For this review, take the finished solid that the model builds, in its own axes (mm). A direction names the side the tool comes from. Coordinates: 2 decimals unless noted, no trailing zeros. Loops run counter-clockwise (first coordinate to the right, second up) from the corner with the lowest first, then second, coordinate; pieces in that order, holes last. Notation, with made-up numbers: (25, 28.25) -> (40, 28.25) arc R30 ccw to (40, 56.25) -> close; hole circle Ø10 at (-3, -38.5). An arc over 180 degrees is marked (long way). One line per item, written item: value.
from build123d import *

# Parameters (mm, degrees)
EXTRUDE_1_DEPTH     = 3
SKETCH_2_W          = 12
SKETCH_2_H          = 12
EXTRUDE_2_DEPTH     = 3.5
SKETCH_3_R          = 4.05
EXTRUDE_3_DEPTH     = 15
CUT_EXTRUDE_1_REACH = 58.993
SKETCH_4_R          = 1.4


with BuildPart() as part:
    # Sketch 1 → Extrude 1 (new body)
    with BuildSketch(Plane(origin=(0, 0, 0), x_dir=(0, 0, -1), z_dir=(1, 0, 0))):
        Polygon((-35, -10), (-35, -41), (0, -41), (0, 41), (-35, 41), (-35, 10), (-10, 10), (-10, -10), align=None)
    extrude(amount=EXTRUDE_1_DEPTH)

    # Sketch 2 → Extrude 2 (add)
    with BuildSketch(Plane(origin=(3, 0, 0), x_dir=(0, 0, -1), z_dir=(1, 0, 0))):
        with Locations((-21, -33.5)):
            Rectangle(SKETCH_2_W, SKETCH_2_H)
    extrude_2 = extrude(amount=EXTRUDE_2_DEPTH)

    # Sketch 3 → Extrude 3 (add)
    with BuildSketch(Plane(origin=(6.5, 0, 0), x_dir=(0, 0, -1), z_dir=(1, 0, 0))):
        with Locations((-21, -33.5)):
            Circle(SKETCH_3_R)
    extrude_3 = extrude(amount=EXTRUDE_3_DEPTH)

    # Mirror 1: Extrude 2, Extrude 3 across plane
    add(extrude_2.mirror(Plane.ZX))
    add(extrude_3.mirror(Plane.ZX))

    # Sketch 4 → Cut-Extrude 1 (cut, up to next)
    with BuildSketch(Plane(origin=(3, 0, 0), x_dir=(0, 0, -1), z_dir=(1, 0, 0)), mode=Mode.PRIVATE) as cut_extrude_1_sk1:
        with Locations((-30, -21)):
            Circle(SKETCH_4_R)
    cut_extrude_1_tool1 = extrude(cut_extrude_1_sk1.sketch, amount=-CUT_EXTRUDE_1_REACH, mode=Mode.PRIVATE) & part.part
    # Sketch 4 → Cut-Extrude 1 (cut, up to next)
    with BuildSketch(Plane(origin=(3, 0, 0), x_dir=(0, 0, -1), z_dir=(1, 0, 0)), mode=Mode.PRIVATE) as cut_extrude_1_sk2:
        with Locations((-5, -36)):
            Circle(SKETCH_4_R)
    cut_extrude_1_tool2 = extrude(cut_extrude_1_sk2.sketch, amount=-CUT_EXTRUDE_1_REACH, mode=Mode.PRIVATE) & part.part
    cut_extrude_1_1 = cut_extrude_1_tool1.solids().sort_by_distance((3, -21, 30))[0]
    add(cut_extrude_1_1, mode=Mode.SUBTRACT)
    cut_extrude_1_2 = cut_extrude_1_tool2.solids().sort_by_distance((3, -36, 5))[0]
    add(cut_extrude_1_2, mode=Mode.SUBTRACT)
    cut_extrude_1 = cut_extrude_1_1 + cut_extrude_1_2  # Cut-Extrude 1 as one shape, for the pattern or mirror that repeats it

    # Mirror 2: Cut-Extrude 1 across plane
    add(cut_extrude_1.mirror(Plane.ZX), mode=Mode.SUBTRACT)


solid = part.part
1. Insertion check: pin 1 Ø1.5 at (x, y) = (18.5, -30) entering from -Z; pin 2 Ø4 at (y, z) = (19, 5.5) entering from +X; pin 3 Ø8 at (y, z) = (8, 30.5) entering from -X; pin 4 Ø1.8 at (x, z) = (4.5, 23.5) entering from +Y. Each pin has a flat end and moves straight along its axis. Give the tip position at first contact, or say it passes through.
Return value:
pin 1: stops at z = 18.03
pin 2: stops at x = 3
pin 3: stops at x = 0
pin 4: stops at y = 39.5
2. The part is to be moulded in two halves that separate along Y. For faces 5 (the flat face through (5, 39.5, 21)), 6 (the flat face through (1, -1, 0)), 7 (the flat face through (6.5, -29, 21)), 8 (the flat face through (5, 27.5, 21)), say which applies: pulls with the +Y half, pulls with the -Y half, needs draft (parallel to the pull), parting line crosses it, or undercut.
Return value:
face 5: pulls with the +Y half
face 6: needs draft
face 7: undercut
face 8: undercut
3. Take a section at C-C, the plane z = 5. Give the boundary of the cut face in (x, y).
Return value:
outline: (0, -41) -> (3, -41) -> (3, -37.4) -> (0, -37.4) -> close; (0, -34.6) -> (3, -34.6) -> (3, 34.6) -> (0, 34.6) -> close; (0, 37.4) -> (3, 37.4) -> (3, 41) -> (0, 41) -> close
4. Take a section at D-D, the plane y = 33.5. Give the boundary of the cut face in (x, z).
Return value:
outline: (0, 0) -> (3, 0) -> (3, 15) -> (6.5, 15) -> (6.5, 16.95) -> (21.5, 16.95) -> (21.5, 25.05) -> (6.5, 25.05) -> (6.5, 27) -> (3, 27) -> (3, 35) -> (0, 35) -> close
5. Take a section at A-A, the plane z = 14. Give the boundary of the cut face in (x, y).
Return value:
outline: (0, -41) -> (3, -41) -> (3, -10) -> (0, -10) -> close; (0, 10) -> (3, 10) -> (3, 41) -> (0, 41) -> close
6. For faces 1 (the flat face through (1, -10, 22)), 2 (the flat face through (5, -34, 15)), 3 (the flat face through (5, -27.5, 21)), 4 (the flat face through (6.5, 29, 21)), list the 3-axis set-ups (+Z, -Z, +X, -X, +Y, -Y) from which the entire face can be reached by the end or side of a thin tool; tool diameter is ignored.
Return value:
face 1: +Z, +X, -X
face 2: -Z, +X, +Y, -Y
face 3: +Z, -Z, +X
face 4: +X
7. Take a section at B-B, the plane y = -21. Give the boundary of the cut face in (x, z).
Return value:
outline: (0, 0) -> (3, 0) -> (3, 28.6) -> (0, 28.6) -> close; (0, 31.4) -> (3, 31.4) -> (3, 35) -> (0, 35) -> close
8. To check wall thickness, follow probe 1 along Y at (x, z) = (1.9, 5); probe 2 along Y at (x, z) = (0.95, 30); probe 3 along Z at (x, y) = (1.35, 36). State the ranges of each line that lie inside material, in increasing order. Write a range as from..to.
Return value:
probe 1: y = -41..-37.4, -34.6..34.6, 37.4..41
probe 2: y = -41..-22.4, -19.6..-10, 10..19.6, 22.4..41
probe 3: z = 0..3.6, 6.4..35
